Geometry: final body of the model. Coordinates: model frame, mm. A direction names the side the tool comes from. Coordinates: 2 decimals unless noted, no trailing zeros. Order: outer loops, then holes, each group sorted by start corner. A loop starts at its lowest first (then second) coordinate and runs counter-clockwise, first axis right, second up. Notation, with made-up numbers: M -4.75,41.5 L 53.25,41.5 A17 cw 53.25,74.5 Z; hole C 59.5,-22.5 d5. An arc over 180 degrees is marked long. Write item = value, one per line.
Autodesk Inventor part; units mm, degrees
ref_plane "YZ Plane" through (0, 0, 0) normal (1, 0, 0) x (0, 1, 0)
ref_plane "XZ Plane" through (0, 0, 0) normal (0, 1, 0) x (-1, 0, 0)
ref_plane "XY Plane" through (0, 0, 0) normal (0, 0, 1) x (1, 0, 0)
sketch "Sketch1" plane through (0, 0, 0) normal (0, 0, 1) x (1, 0, 0)
  line L0 (508.715, -158.715) -> (-5.715, -158.715) construction
  line L1 (-5.715, -158.715) -> (-5.715, 8.715)
  line L2 (-5.715, 8.715) -> (508.715, 8.715) construction
  line L3 (508.715, 8.715) -> (508.715, -158.715)
  line L4 (-5.715, 8.715) -> (-5.715, 48.715)
  line L5 (-5.715, 48.715) -> (44.285, 48.715)
  arc A0 (99.6722, 45.6378) -> (44.285, 48.715) centre (44.285, -451.285) ccw
  line L6 (99.6722, 45.6378) -> (403.3278, 11.7922)
  arc A1 (403.3278, 11.7922) -> (458.715, 8.715) centre (458.715, 508.715) ccw
  line L7 (458.715, 8.715) -> (508.715, 8.715)
  line L8 (-5.715, -158.715) -> (-5.715, -198.715)
  line L9 (-5.715, -198.715) -> (44.285, -198.715)
  arc A2 (44.285, -198.715) -> (99.6722, -195.6378) centre (44.285, 301.285) ccw
  line L10 (99.6722, -195.6378) -> (403.3278, -161.7922)
  arc A3 (458.715, -158.715) -> (403.3278, -161.7922) centre (458.715, -658.715) ccw
  line L11 (458.715, -158.715) -> (508.715, -158.715)
  point P0 (0, 0)
  point P1 (0, 5.715)
  point P2 (505.715, -158.715)
  point P3 (505.715, 8.715)
  point P4 (-5.715, 5.715)
  dimension "d0" = 3
  dimension "d2" = 500
  dimension "d3" = 50
  dimension "d4" = 40
extrude "Extrusion1" add sketch "Sketch1" along normal blind 5.715
fillet "Fillet1" radius 3 2 edges at (508.715, 8.715, 2.8575) (508.715, -158.715, 2.8575)
sketch "Sketch2" plane through (0, 0, 5.715) normal (0, 0, 1) x (1, 0, 0)
  line L0 (24.6425, 0) -> (34.6425, 0)
  line L1 (34.6425, 5.715) -> (34.6425, 0)
  line L2 (34.6425, 5.715) -> (24.6425, 5.715)
  line L3 (24.6425, 5.715) -> (24.6425, 0)
  line L4 (59.6425, 0) -> (69.6425, 0)
  line L5 (69.6425, 5.715) -> (69.6425, 0)
  line L6 (69.6425, 5.715) -> (59.6425, 5.715)
  line L7 (59.6425, 5.715) -> (59.6425, 0)
  line L8 (224.6425, 0) -> (234.6425, 0)
  line L9 (234.6425, 5.715) -> (234.6425, 0)
  line L10 (234.6425, 5.715) -> (224.6425, 5.715)
  line L11 (224.6425, 5.715) -> (224.6425, 0)
  line L12 (259.6425, 0) -> (269.6425, 0)
  line L13 (269.6425, 5.715) -> (269.6425, 0)
  line L14 (269.6425, 5.715) -> (259.6425, 5.715)
  line L15 (259.6425, 5.715) -> (259.6425, 0)
  line L16 (424.6425, 0) -> (434.6425, 0)
  line L17 (434.6425, 5.715) -> (434.6425, 0)
  line L18 (434.6425, 5.715) -> (424.6425, 5.715)
  line L19 (424.6425, 5.715) -> (424.6425, 0)
  line L20 (459.6425, 0) -> (469.6425, 0)
  line L21 (469.6425, 5.715) -> (469.6425, 0)
  line L22 (469.6425, 5.715) -> (459.6425, 5.715)
  line L23 (459.6425, 5.715) -> (459.6425, 0)
  line L24 (500, -40) -> (500, -30)
  line L25 (505.715, -40) -> (500, -40)
  line L26 (505.715, -30) -> (505.715, -40)
  line L27 (505.715, -30) -> (500, -30)
  line L28 (500, -120) -> (500, -110)
  line L29 (505.715, -120) -> (500, -120)
  line L30 (505.715, -110) -> (505.715, -120)
  line L31 (505.715, -110) -> (500, -110)
  line L32 (459.6425, -155.715) -> (469.6425, -155.715)
  line L33 (469.6425, -150) -> (469.6425, -155.715)
  line L34 (469.6425, -150) -> (459.6425, -150)
  line L35 (459.6425, -150) -> (459.6425, -155.715)
  line L36 (424.6425, -155.715) -> (434.6425, -155.715)
  line L37 (434.6425, -150) -> (434.6425, -155.715)
  line L38 (434.6425, -150) -> (424.6425, -150)
  line L39 (424.6425, -150) -> (424.6425, -155.715)
  line L40 (259.6425, -155.715) -> (269.6425, -155.715)
  line L41 (269.6425, -150) -> (269.6425, -155.715)
  line L42 (269.6425, -150) -> (259.6425, -150)
  line L43 (259.6425, -150) -> (259.6425, -155.715)
  line L44 (224.6425, -155.715) -> (234.6425, -155.715)
  line L45 (234.6425, -150) -> (234.6425, -155.715)
  line L46 (234.6425, -150) -> (224.6425, -150)
  line L47 (224.6425, -150) -> (224.6425, -155.715)
  line L48 (59.6425, -155.715) -> (69.6425, -155.715)
  line L49 (69.6425, -150) -> (69.6425, -155.715)
  line L50 (69.6425, -150) -> (59.6425, -150)
  line L51 (59.6425, -150) -> (59.6425, -155.715)
  line L52 (24.6425, -155.715) -> (34.6425, -155.715)
  line L53 (34.6425, -150) -> (34.6425, -155.715)
  line L54 (34.6425, -150) -> (24.6425, -150)
  line L55 (24.6425, -150) -> (24.6425, -155.715)
  line L56 (34.6425, 2.8575) -> (59.6425, 2.8575) construction
  circle A0 centre (47.1425, 2.8575) radius 1.5
  line L57 (234.6425, 2.8575) -> (259.6425, 2.8575) construction
  circle A1 centre (247.1425, 2.8575) radius 1.5
  line L58 (434.6425, 2.8575) -> (459.6425, 2.8575) construction
  circle A2 centre (447.1425, 2.8575) radius 1.5
  line L59 (502.8575, -40) -> (502.8575, -110) construction
  circle A3 centre (502.8575, -75) radius 1.5
  line L60 (434.6425, -152.8575) -> (459.6425, -152.8575) construction
  circle A4 centre (447.1425, -152.8575) radius 1.5
  line L61 (234.6425, -152.8575) -> (259.6425, -152.8575) construction
  circle A5 centre (247.1425, -152.8575) radius 1.5
  line L62 (34.6425, -152.8575) -> (59.6425, -152.8575) construction
  circle A6 centre (47.1425, -152.8575) radius 1.5
  point P0 (0, 0)
  dimension "d8" = 3
  dimension "d10" = 3
  dimension "d11" = 3
  dimension "d12" = 3
  dimension "d13" = 3
  dimension "d14" = 3
  dimension "d15" = 3
extrude "Extrusion2" cut sketch "Sketch2" against normal through all
sketch "Sketch3" plane through (0, 0, 5.715) normal (0, 0, 1) x (1, 0, 0)
  line L0 (75, -30) -> (75, -40)
  line L1 (75, -30) -> (69.285, -30)
  line L2 (69.285, -40) -> (69.285, -30)
  line L3 (75, -40) -> (69.285, -40)
  line L4 (75, -110) -> (75, -120)
  line L5 (75, -110) -> (69.285, -110)
  line L6 (69.285, -120) -> (69.285, -110)
  line L7 (75, -120) -> (69.285, -120)
  line L8 (72.1425, -40) -> (72.1425, -110)
  circle A0 centre (72.1425, -75) radius 1.5
  point P0 (0, 0)
  dimension "d18" = 3
extrude "Extrusion3" cut sketch "Sketch3" against normal through all
sketch "Sketch4" plane through (0, 0, 5.715) normal (0, 0, 1) x (1, 0, 0)
  circle A0 centre (502.8575, -75) radius 1.5
  line L0 (508.715, -155.715) -> (508.715, 5.715)
  line L1 (458.715, -158.715) -> (505.715, -158.715)
  line L2 (453.715, -110) -> (453.715, -40)
  arc A1 (483.715, -40) -> (453.715, -40) centre (468.715, -40) ccw
  line L3 (483.715, -40) -> (483.715, -110)
  arc A2 (453.715, -110) -> (483.715, -110) centre (468.715, -110) ccw
  point P0 (0, 0)
  point P1 (483.715, -75)
  dimension "d22" = 70
  dimension "d25" = 15
  dimension "d26" = 25
extrude "Extrusion4" cut sketch "Sketch4" against normal through all contours L2 A1 L3 A2
properties part number "SIDE PLATE"
1) Mould query, pull axis Y, two halves, no side actions, for faces 3 (the face through (468.385, -124.996, 2.898)), 4 (the face through (249.374, -178.952, 2.817)), 5 (the face through (191, -73, 5.715)). Classes: pulls with the +Y half, pulls with the -Y half, needs draft (parallel to the pull), parting line crosses it, or undercut.
Numbers:
face_3 = undercut
face_4 = pulls with the -Y half
face_5 = needs draft
2) Section C-C, the plane x = 169. Return loops of the section in (y, z) (3 decimals), and give its area (3 significant figures).
Numbers:
outline = M -187.91,0 L 37.91,0 L 37.91,5.715 L -187.91,5.715 Z
area = 1,290 mm²
3) Line query: L1, parallel to X at y = -100.5, z = 3.95 (3 decimals); L2, parallel to Y at x = 230.5, z = 3.75 (3 decimals); L3, parallel to Y at x = 63, z = 2.6 (3 decimals). Output: solid intervals per line, ascending.
Numbers:
L1 = -5.715 to 453.715, 483.715 to 508.715
L2 = -181.056 to -155.715, -150 to 0, 5.715 to 31.056
L3 = -198.365 to -155.715, -150 to 0, 5.715 to 48.365
4) Section A-A, the plane z = 2.15. Give the number of separate pieces and of enclosed holes in the cut face, and give its area (3 significant figures).
Numbers:
separate_pieces = 1
enclosed_holes = 25
area = 103,000 mm²
5) Pin query (flat end, axial travel): pin 1 (1.7 mm diameter, centred on x = 503.5, z = 3.5, fed in from -Y) (3 decimals). Return the tip coordinate at first contact, or that it passes through.
Numbers:
pin_1 = -158.715
6) Set-up query: faces 1 (the face through (249.374, 28.952, 2.817)), 2 (the face through (469.045, -25.004, 2.898)). Return all of +Z, -Z, +X, -X, +Y, -Y with unobstructed straight access to the full face (end or side cutting, diameter ignored); none if empty.
Numbers:
face_1 = +Z, -Z, +X, +Y
face_2 = +Z, -Z
7) Section B-B, the plane x = 377.5. Return loops of the section in (y, z) (3 decimals), and give its area (3 significant figures).
Numbers:
outline = M -164.671,0 L 14.671,0 L 14.671,5.715 L -164.671,5.715 Z
area = 1,020 mm²
